Build history of the part. All positions in model axes, mm. A direction names the side the tool comes from. Coordinates: 2 decimals unless noted, no trailing zeros. Order: outer loops, then holes, each group sorted by start corner. A loop starts at its lowest first (then second) coordinate and runs counter-clockwise, first axis right, second up. Notation, with made-up numbers: (19, 83.5) - (50, 83.5) arc R29 cw to (50, 103.5) - close; hole circle Ø10 at (50, 48). An arc over 180 degrees is marked (long way). One line per item, written item: value.
Autodesk Inventor part; units mm, degrees
ref_plane "Work Plane1" through (0, 50, 100) normal (0, 1, 0) x (-1, 0, 0)
ref_plane "YZ Plane" through (0, 0, 0) normal (1, 0, 0) x (0, 1, 0)
ref_plane "XY Plane" through (0, 0, 0) normal (0, 0, 1) x (1, 0, 0)
sketch "Sketch1" plane through (0, 0, 0) normal (1, 0, 0) x (0, 1, 0)
  line L0 (50, -100) -> (-50, -100) construction
  line L1 (-50, -100) -> (-50, 100) construction
  line L2 (-50, 100) -> (50, 100) construction
  line L3 (50, 100) -> (50, -100) construction
  line L4 (50, -100) -> (-50, 100) construction
  line L5 (-50, -100) -> (50, 100) construction
  line L6 (50, 100) -> (-40, 100)
  arc A0 (-40, 100) -> (-50, 90) centre (-40, 90) ccw
  line L7 (50, -100) -> (-40, -100)
  arc A1 (-50, -90) -> (-40, -100) centre (-40, -90) ccw
  line L8 (-50, -90) -> (-50, 90)
  point P0 (0, 0)
  dimension "d0" = 100
  dimension "d1" = 200
  dimension "d2" = 90
  dimension "d3" = 90
ref_plane "Work Plane1" through (0, 50, 100) normal (0, 1, 0) x (-1, 0, 0)
sketch "Sketch2" plane through (0, 50, 100) normal (0, 1, 0) x (-1, 0, 0)
  line L0 (56, 0) -> (-194, 0)
  line L1 (-194, 0) -> (-194, -3)
  line L2 (-194, -3) -> (56, -3)
  line L3 (56, -3) -> (56, 0)
  point P0 (0, -100)
  dimension "d4" = 250
  dimension "d5" = 3
sweep "Sweep1" add profiles "Sketch2" path "Sketch1"
sketch "Sketch3" plane through (-56, -47, 90) normal (0, 1, 0) x (1, 0, 0)
  circle A0 centre (50, 90) radius 30
  line L0 (175, 25) -> (230, 25)
  line L1 (230, 25) -> (230, 50)
  line L2 (230, 50) -> (175, 50)
  line L3 (175, 50) -> (175, 25)
  line L4 (250, 0) -> (250, 180)
  line L5 (0, 0) -> (250, 0)
  line L6 (56, 90) -> (50, 90) construction
  line L7 (50, 90) -> (250, 90) construction
  line L8 (175, 155) -> (230, 155)
  line L9 (230, 155) -> (230, 130)
  line L10 (230, 130) -> (175, 130)
  line L11 (175, 130) -> (175, 155)
  line L12 (0, 0) -> (0, 180)
  circle A1 centre (120, 90) radius 5
  dimension "d8" = 60
  dimension "d10" = 55
  dimension "d11" = 25
  dimension "d12" = 20
  dimension "d13" = 25
  dimension "d25" = 50
  dimension "d26" = 10
  dimension "d27" = 120
extrude "Extrusion1" cut sketch "Sketch3" against normal through all
sketch "Sketch4" plane through (-56, 50, 100) normal (0, 0, 1) x (1, 0, 0)
  line L0 (0, 0) -> (0, -90)
  line L1 (250, -90) -> (0, -90)
  point P0 (56, -50)
  point P1 (50, -80)
  dimension "d16" = 50
  dimension "d17" = 10
hole "Hole1" at (-6, -30, 100) direction (0, 0, -1) diameter 3 end through all
equation "\"d3\" = d2"
properties material "PMMA Plastic"
1. Probe line 1 along X through (y, z) = (-48.9, 0); line 2 along Z through (x, y) = (128.5, 22.5); line 3 along X through (y, z) = (-30, 99.35). List the from-to ranges inside material, lowest first.
Values found:
line 1: x = -56 to -36, 24 to 59, 69 to 194
line 2: z = -100 to -97, 97 to 100
line 3: x = -56 to -7.5, -4.5 to 194
2. Two-plate mould, pull along Z, no slides. Class faces 3 (the face through (67, 4, 100)), 4 (the face through (70.75, -47.15, -96.99)), 5 (the face through (68.619, -48.479, 1.915)), 6 (the face through (21.712, -48.479, 11.49)): pulls with the +Z half, pulls with the -Z half, needs draft (parallel to the pull), parting line crosses it, or undercut.
Values found:
face 3: pulls with the +Z half
face 4: pulls with the -Z half
face 5: undercut
face 6: undercut
3. Band-saw the part on C-C, the plane z = -51. Give the cut face in (x, y), and give its area (3 significant figures).
Values found:
outline: (-56, -50) - (119, -50) - (119, -47) - (-56, -47) - close; (174, -50) - (194, -50) - (194, -47) - (174, -47) - close
area: 585 mm2
4. Band-saw the part on B-B, the plane x = 64. Give the cut face in (y, z).
Values found:
outline: (-50, -90) arc R10 ccw to (-40, -100) - (50, -100) - (50, -97) - (-40, -97) arc R7 cw to (-47, -90) - (-47, -5) - (-50, -5) - close; (-50, 5) - (-47, 5) - (-47, 90) arc R7 cw to (-40, 97) - (50, 97) - (50, 100) - (-40, 100) arc R10 ccw to (-50, 90) - close
5. Band-saw the part on A-A, the plane z = 0. Give the cut face in (x, y).
Values found:
outline: (-56, -50) - (-36, -50) - (-36, -47) - (-56, -47) - close; (24, -50) - (59, -50) - (59, -47) - (24, -47) - close; (69, -50) - (194, -50) - (194, -47) - (69, -47) - close
6. Band-saw the part on D-D, the plane y = 39. Give the cut face in (x, z).
Values found:
outline: (-56, -100) - (194, -100) - (194, -97) - (-56, -97) - close; (-56, 97) - (194, 97) - (194, 100) - (-56, 100) - close
7. 3-axis set-ups, long thin cutter, end or side, ignore diameter. For faces 1 (the face through (67.2, -44.9, -95)), 2 (the face through (-56, -48, 0)): which of +Z, -Z, +X, -X, +Y, -Y reach the whole face in a straight line?
Values found:
face 1: +X, -X, +Y
face 2: +Z, -Z, -X, +Y, -Y
8. Flat gauge pins, fed straight in: P1, Ø4, axis at x = -6, y = -30, coming from the +Z side; P2, Ø1.5, axis at x = 152, y = -49, coming from the +Z side; P3, Ø1.5, axis at x = 50.5, z = -42, coming from the +Y side; P4, Ø0.9, axis at x = 147.5, y = -48, coming from the +Z side. Where does each tip first touch, or does it go through?
Values found:
P1: stops at z = 100
P2: stops at z = 95.65
P3: stops at y = -47
P4: stops at z = 96.56
